Can you work these out from the model? Positions are in its coordinate system, mm. A direction names the side the tool comes from. Round coordinates to 2 decimals unless told otherwise and drop trailing zeros. Write each loop counter-clockwise with the first axis right and the second up, starting at its lowest first coordinate (ties: lowest second). Pieces come first, ordered by that corner, then holes. Notation, with made-up numbers: (67.25, 23) -> (100.25, 23) arc R19 ccw to (100.25, 36) -> close; hole circle Ø10 at (43, -28.75). An arc over 180 degrees is marked (long way). Write item = value, one per line. Start each with the question number.
1) Imagine slicing it at D-D, the plane z = 14. Please give me the cut outline in (x, y).
2) I'm going to push flat-ended pins straight in: pin 1 (0.6 mm diameter, centred on y = 1.5, z = -14, fed in from +X); pin 2 (0.6 mm diameter, centred on x = 12.5, y = 1.5, fed in from +Z). Where does each tip first touch, or does it pass through?
3) Imagine slicing it at B-B, the plane x = 0. Please give me the cut outline in (y, z).
4) Imagine slicing it at C-C, the plane y = 0.45. State how many separate pieces and enclosed holes the cut face has, then the cut area to 3 significant figures.
5) Imagine slicing it at A-A, the plane z = 0. Please give me the cut outline in (x, y).
6) Thinking about a two-plate mould opening in Z: for faces 4 (the face through (-0.08, 0.99, 20.05)), 5 (the face through (-15.06, 0.99, -0.16)), 6 (the face through (0, 2, -2)), which applies, +Z half, -Z half, draft (parallel to the pull), parting line (faces both ways), or undercut?
7) For faces 1 (the face through (13, 1, -3.75)), 2 (the face through (3.75, 1, 13)), 3 (the face through (-3.75, 1, -13)), which set-ups out of +Z, -Z, +X, -X, +Y, -Y let a thin tool reach every point of the face, with its end or its side?
8) If I drill on line 1 (X direction, y = 1.05, z = 0); line 2 (Z direction, x = 13, y = 1.3); line 3 (X direction, y = 0.7, z = 16.3), over which ranges is the centre line in solid material (lowest first)?
from build123d import *

# Parameters (mm, degrees)
SKETCH_1_R      = 1.25
EXTRUDE_1_DEPTH = 2


with BuildPart() as part:
    # 草圖1 → 填料-伸長1 (new body)
    with BuildSketch(Plane(origin=(0, 0, 0), x_dir=(1, 0, 0), z_dir=(0, 1, 0))):
        with BuildLine():
            Line((-3.75, 16.3), (-3.75, 9.75))
            ThreePointArc((-3.75, 9.75), (-5.507359313, 5.507359313), (-9.75, 3.75))
            Line((-9.75, 3.75), (-16.3, 3.75))
            ThreePointArc((-16.3, 3.75), (-20.05, 0), (-16.3, -3.75))
            Line((-16.3, -3.75), (-9.75, -3.75))
            ThreePointArc((-9.75, -3.75), (-5.507359313, -5.507359313), (-3.75, -9.75))
            Line((-3.75, -9.75), (-3.75, -16.3))
            ThreePointArc((-3.75, -16.3), (0, -20.05), (3.75, -16.3))
            Line((3.75, -16.3), (3.75, -9.75))
            ThreePointArc((3.75, -9.75), (5.507359313, -5.507359313), (9.75, -3.75))
            Line((9.75, -3.75), (16.3, -3.75))
            ThreePointArc((16.3, -3.75), (20.05, 0), (16.3, 3.75))
            Line((16.3, 3.75), (9.75, 3.75))
            ThreePointArc((9.75, 3.75), (5.507359313, 5.507359313), (3.75, 9.75))
            Line((3.75, 9.75), (3.75, 16.3))
            ThreePointArc((3.75, 16.3), (0, 20.05), (-3.75, 16.3))
        make_face()
        with Locations(Location((0, 16.3, 0), (0, 0, 270))):
            Circle(SKETCH_1_R, mode=Mode.SUBTRACT)
        with Locations(Location((-16.3, 0, 0), (0, 0, 270))):
            Circle(SKETCH_1_R, mode=Mode.SUBTRACT)
        with Locations(Location((0, -16.3, 0), (0, 0, 270))):
            Circle(SKETCH_1_R, mode=Mode.SUBTRACT)
        with Locations(Location((16.3, 0, 0), (0, 0, 270))):
            Circle(SKETCH_1_R, mode=Mode.SUBTRACT)
        with Locations(Location((0, 9.5, 0), (0, 0, 270))):
            Circle(SKETCH_1_R, mode=Mode.SUBTRACT)
        with Locations(Location((-8, 0, 0), (0, 0, 270))):
            Circle(SKETCH_1_R, mode=Mode.SUBTRACT)
        with Locations(Location((0, -9.5, 0), (0, 0, 270))):
            Circle(SKETCH_1_R, mode=Mode.SUBTRACT)
        with Locations(Location((8, 0, 0), (0, 0, 270))):
            Circle(SKETCH_1_R, mode=Mode.SUBTRACT)
    extrude(amount=EXTRUDE_1_DEPTH)


solid = part.part
Reported:
q1.outline = (-3.75, 0) -> (3.75, 0) -> (3.75, 2) -> (-3.75, 2) -> close
q2.pin_1 = 3.75
q2.pin_2 = 3.75
q3.outline = (0, -20.05) -> (2, -20.05) -> (2, -17.55) -> (0, -17.55) -> close; (0, -15.05) -> (2, -15.05) -> (2, -10.75) -> (0, -10.75) -> close; (0, -8.25) -> (2, -8.25) -> (2, 8.25) -> (0, 8.25) -> close; (0, 10.75) -> (2, 10.75) -> (2, 15.05) -> (0, 15.05) -> close; (0, 17.55) -> (2, 17.55) -> (2, 20.05) -> (0, 20.05) -> close
q4.separate_pieces = 1
q4.enclosed_holes = 8
q4.area = 513 mm²
q5.outline = (-20.05, 0) -> (-17.55, 0) -> (-17.55, 2) -> (-20.05, 2) -> close; (-15.05, 0) -> (-9.25, 0) -> (-9.25, 2) -> (-15.05, 2) -> close; (-6.75, 0) -> (6.75, 0) -> (6.75, 2) -> (-6.75, 2) -> close; (9.25, 0) -> (15.05, 0) -> (15.05, 2) -> (9.25, 2) -> close; (17.55, 0) -> (20.05, 0) -> (20.05, 2) -> (17.55, 2) -> close
q6.face_4 = +Z half
q6.face_5 = undercut
q6.face_6 = draft
q7.face_1 = -Z, +X, +Y, -Y
q7.face_2 = +Z, +X, +Y, -Y
q7.face_3 = -Z, -X, +Y, -Y
q8.line_1 = -20.05 to -17.55, -15.05 to -9.25, -6.75 to 6.75, 9.25 to 15.05, 17.55 to 20.05
q8.line_2 = -3.75 to 3.75
q8.line_3 = -3.75 to -1.25, 1.25 to 3.75
